```python
from build123d import *

# Parameters (mm, degrees)
SKETCH5_R           = 1.65
SKETCH5_R_2         = 12.7
BOSS_EXTRUDE1_DEPTH = 3.175


with BuildPart() as part:
    # Sketch5 → Boss-Extrude1 (new body)
    with BuildSketch(Plane.XY):
        Polygon((47.124604737, -7.452255775), (30.614604737, -7.452255775), (30.614604737, 71.287744225), (47.124604737, 71.287744225), (47.124604737, 149.14592508), (30.614604737, 149.14592508), (30.614604737, 227.88592508), (47.124604737, 227.88592508), (47.124604737, 249.558730102), (-36.302449898, 249.558730102), (-36.302449898, 234.650730102), (-24.302449898, 234.650730102), (-24.302449898, 227.030730102), (-36.302449898, 227.030730102), (-56.302449898, 227.030730102), (-68.302449898, 227.030730102), (-68.302449898, 234.650730102), (-56.302449898, 234.650730102), (-56.302449898, 249.558730102), (-154.402428268, 249.558730102), (-154.402428268, 234.650730102), (-142.402428268, 234.650730102), (-142.402428268, 227.030730102), (-154.402428268, 227.030730102), (-174.402428268, 227.030730102), (-186.402428268, 227.030730102), (-186.402428268, 234.650730102), (-174.402428268, 234.650730102), (-174.402428268, 249.558730102), (-252.849395263, 249.558730102), (-252.849395263, 227.88592508), (-236.339395263, 227.88592508), (-236.339395263, 149.14592508), (-252.849395263, 149.14592508), (-252.849395263, 71.287744225), (-236.339395263, 71.287744225), (-236.339395263, -7.452255775), (-252.849395263, -7.452255775), (-252.849395263, -30.349269898), (47.124604737, -30.349269898), align=None)
        with Locations((39.94351791, -22.890690042)):
            Circle(SKETCH5_R, mode=Mode.SUBTRACT)
        with Locations((-17.05648209, -22.890690042)):
            Circle(SKETCH5_R, mode=Mode.SUBTRACT)
        with Locations((-74.05648209, -22.890690042)):
            Circle(SKETCH5_R, mode=Mode.SUBTRACT)
        with Locations((-131.05648209, -22.890690042)):
            Circle(SKETCH5_R, mode=Mode.SUBTRACT)
        with Locations((-188.05648209, -22.890690042)):
            Circle(SKETCH5_R, mode=Mode.SUBTRACT)
        with Locations((-245.05648209, -22.890690042)):
            Circle(SKETCH5_R, mode=Mode.SUBTRACT)
        with Locations((39.94351791, 242.101620414)):
            Circle(SKETCH5_R, mode=Mode.SUBTRACT)
        with Locations((-17.05648209, 242.101620414)):
            Circle(SKETCH5_R, mode=Mode.SUBTRACT)
        with Locations((-74.05648209, 242.101620414)):
            Circle(SKETCH5_R, mode=Mode.SUBTRACT)
        with Locations((-131.05648209, 242.101620414)):
            Circle(SKETCH5_R, mode=Mode.SUBTRACT)
        with Locations((-188.05648209, 242.101620414)):
            Circle(SKETCH5_R, mode=Mode.SUBTRACT)
        with Locations((-245.05648209, 242.101620414)):
            Circle(SKETCH5_R, mode=Mode.SUBTRACT)
        with Locations((-102.862395263, 184.854342805)):
            Circle(SKETCH5_R_2, mode=Mode.SUBTRACT)
        with Locations((-102.862395263, 45.850730102)):
            Circle(SKETCH5_R_2, mode=Mode.SUBTRACT)
    extrude(amount=BOSS_EXTRUDE1_DEPTH)


solid = part.part
```
Work out the finished part from the listing and answer in its coordinate system (mm). Round coordinates to 2 decimals unless told otherwise and drop trailing zeros. Write each loop counter-clockwise with the first axis right and the second up, starting at its lowest first coordinate (ties: lowest second). Pieces come first, ordered by that corner, then holes. Notation, with made-up numbers: (26, 81.25) - (62, 81.25) arc R19 cw to (62, 99.25) - close; hole circle Ø3 at (-31.5, -13.5). An arc over 180 degrees is marked (long way). Return JSON: item names as keys, results as strings. Group by question number.
Q1. The part is cut by section A-A on y = 181.5. Write down the section's boundary in (x, z) (3 decimals).
Q2. The mould has two halves that part along Y. Classify faces 1 (the flat face through (-105, 112, 0)), 2 (the cylindrical face through (-104.516, 58.443, 1.565)): released by +Y, released by -Y, zero draft, split by the parting line, or undercut.
Q3. The part is cut by section B-B on y = 10.5. Write down the section's boundary in (x, z) (3 decimals), then the cut area to 3 significant figures.
Q4. This flat-tipped pin is pushed along its axis until it touches: pin 1 Ø1.5 at (x, z) = (-50.5, 0.5) entering from +Y. Where does it stop, or does it pass through?
Q5. Find the intervals of material crossed by L1, parallel to Y at x = -176, z = 2.8; L2, parallel to X at y = 17, z = 1.25; L3, parallel to Y at x = -49.5, z = 1.65, in increasing order.
Q6. The part is cut by section C-C on z = 0.7. Count the separate pieces of the cut face and the enclosed holes in it, then the cut area to 3 significant figures.
Solved:
{
 "1": {"outline": "(-236.339, 0) - (-115.111, 0) - (-115.111, 3.175) - (-236.339, 3.175) - close; (-90.613, 0) - (30.615, 0) - (30.615, 3.175) - (-90.613, 3.175) - close"},
 "2": {"face 1": "zero draft", "face 2": "undercut"},
 "3": {"outline": "(-236.339, 0) - (30.615, 0) - (30.615, 3.175) - (-236.339, 3.175) - close", "area": "848 mm²"},
 "4": {"pin 1": "y = 227.03"},
 "5": {"L1": "-30.35 to 227.03, 234.65 to 249.56", "L2": "-236.34 to 30.61", "L3": "-30.35 to 227.03"},
 "6": {"separate pieces": "1", "enclosed holes": "14", "area": "76,400 mm²"}
}
